```python
from build123d import *
from build123d.topology import SkipClean

# Parameters (mm, degrees)
SKETCH1_R          = 13.97
SKETCH1_R_2        = 6.604
STABILIZER_DEPTH   = 1.27
LARGE_START        = 7.9375
SKETCH2_R          = 7.366
SKETCH2_R_2        = 6.604
LARGE_END_DEPTH    = 7.9375
SMALL_START        = 7.9375
SKETCH3_R          = 7.366
SKETCH3_R_2        = 6.096
SMALL_END_DEPTH    = 7.9375
SKETCH5_W          = 3.81
SKETCH5_H          = 13.335
CUT_EXTRUDE1_DEPTH = 31.730063798
SKETCH7_W          = 3.81
SKETCH7_H          = 13.335
CUT_EXTRUDE2_DEPTH = 31.730063798


with BuildPart() as part:
    # Sketch1 → Stabilizer (new body)
    with BuildSketch(Plane(origin=(0, 0, 0), x_dir=(1, 0, 0), z_dir=(0, 1, 0))):
        with Locations(Location((0, 0, 0), (0, 0, 270))):
            Circle(SKETCH1_R)
        with Locations(Location((0, 0, 0), (0, 0, 270))):
            Circle(SKETCH1_R_2, mode=Mode.SUBTRACT)
    extrude(amount=STABILIZER_DEPTH)

    # Sketch2 → Large End (add)
    with SkipClean():  # the faces are left unmerged after this step: merging them gives an invalid solid
        with BuildSketch(Plane(origin=(0, 0, 0), x_dir=(-1, 0, 0), z_dir=(0, -1, 0)).offset(LARGE_START)):
            with Locations(Location((0, 0, 0), (0, 0, 270))):
                Circle(SKETCH2_R)
            with Locations(Location((0, 0, 0), (0, 0, 90))):
                Circle(SKETCH2_R_2, mode=Mode.SUBTRACT)
        extrude(amount=-LARGE_END_DEPTH)

    # Sketch3 → Small End (add)
    with SkipClean():  # the faces are left unmerged after this step: merging them gives an invalid solid
        with BuildSketch(Plane(origin=(0, -7.9375, 0), x_dir=(-1, 0, 0), z_dir=(0, -1, 0)).offset(SMALL_START)):
            with Locations(Location((0, 0, 0), (0, 0, 270))):
                Circle(SKETCH3_R)
            with Locations(Location((0, 0, 0), (0, 0, 90))):
                Circle(SKETCH3_R_2, mode=Mode.SUBTRACT)
        extrude(amount=-SMALL_END_DEPTH)

    # Sketch5 → Cut-Extrude1 (cut, through all)
    with SkipClean():  # the faces are left unmerged after this step: merging them gives an invalid solid
        with BuildSketch(Plane(origin=(0, -15.875, 7.366), x_dir=(1, 0, 0), z_dir=(0, 0, 1))):
            with Locations((0, 9.2075)):
                Rectangle(SKETCH5_W, SKETCH5_H)
        extrude(amount=-CUT_EXTRUDE1_DEPTH, mode=Mode.SUBTRACT)
    add(part.part.scale(1), mode=Mode.REPLACE)  # the faces are merged on a copy

    # Sketch7 → Cut-Extrude2 (cut, through all)
    with BuildSketch(Plane(origin=(7.366, -15.875, 0), x_dir=(0, 0, -1), z_dir=(1, 0, 0))):
        with Locations((0, 9.2075)):
            Rectangle(SKETCH7_W, SKETCH7_H)
    extrude(amount=-CUT_EXTRUDE2_DEPTH, mode=Mode.SUBTRACT)


solid = part.part
```
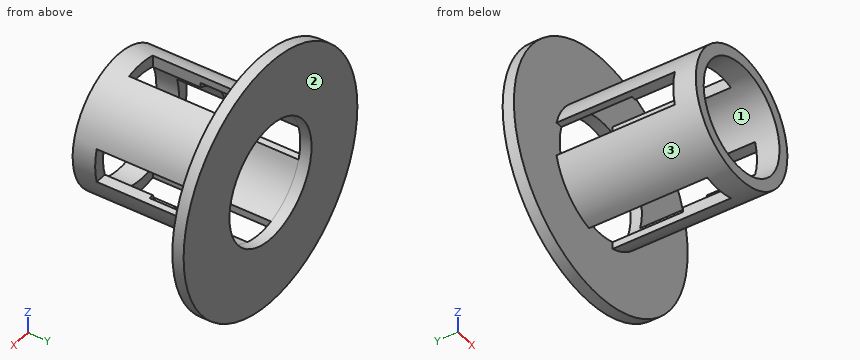
Could you check a few things on this model? Use its own coordinates, in mm. Face numbers are marked on the shaded views. Give positions to 0.01 mm unless a question says otherwise; leave off trailing zeros. Loops run counter-clockwise (first coordinate to the right, second up) from the corner with the lowest first, then second, coordinate; pieces in that order, holes last. Notation, with made-up numbers: (-7.75, 1.25) - (30.25, 1.25) arc R26 cw to (30.25, 17.25) - close; hole circle Ø2 at (-3, 17.25). An arc over 180 degrees is marked (long way). Answer in a Markdown table with one row per item. Add a question column.
Q1. If we section it at D-D (y = -14.5): List the corners of the cut face in (x, z) for me.
Q2. Please list where these lines run through material, in increasing order: L1, parallel to X at y = 1, z = 0; L2, parallel to X at y = -13.75, z = 0. Write a range as from..to.
Q3. If we section it at B-B (x = 0): List the corners of the cut face in (y, z) for me (3 decimals).
Q4. If we section it at C-C (z = 4): List the corners of the cut face in (x, y) for me (1 decimal), plus the area to 3 significant figures.
Q5. We'd pull the mould along Z, two halves only. Please class the marked faces 1, 2 and 3: +Z half, -Z half, draft (parallel to the pull), parting line (faces both ways), or undercut.
Q6. For pin 1 (0.7 mm diameter, centred on x = -6.5, y = -6.5, fed in from -Z); pin 2 (1.3 mm diameter, centred on x = 4.5, z = 4, fed in from +Y); pin 3 (0.7 mm diameter, centred on y = -6.5, z = 6, fed in from -X); pin 4 (8 mm diameter, centred on x = 0, z = 0.5, fed in from +Y), each with a flat end and sliding along its axis, tell me the tip position at first contact or that it passes through.
Q7. If we section it at A-A (y = -3.5): List the corners of the cut face in (x, z) for me (3 decimals), plus the area to 3 significant figures.
The answers:
| question | item | result |
|---|---|---|
| 1 | outline | circle Ø14.73 at (0, 0); hole circle Ø12.19 at (0, 0) |
| 2 | L1 | x = -13.97..-6.6, 6.6..13.97 |
| 2 | L2 | x = -7.37..-6.1, 6.1..7.37 |
| 3 | outline | (-15.875, -7.366) - (-13.335, -7.366) - (-13.335, -6.096) - (-15.875, -6.096) - close; (-15.875, 6.096) - (-13.335, 6.096) - (-13.335, 7.366) - (-15.875, 7.366) - close; (0, -13.97) - (1.27, -13.97) - (1.27, -6.604) - (0, -6.604) - close; (0, 6.604) - (1.27, 6.604) - (1.27, 13.97) - (0, 13.97) - close |
| 4 | outline | (-13.4, 0) - (-6.2, 0) - (-6.2, -15.9) - (-4.6, -15.9) - (-4.6, -7.9) - (-5.3, -7.9) - (-5.3, 1.3) - (-13.4, 1.3) - close; (4.6, -15.9) - (6.2, -15.9) - (6.2, 0) - (13.4, 0) - (13.4, 1.3) - (5.3, 1.3) - (5.3, -7.9) - (4.6, -7.9) - close |
| 4 | area | 60.6 mm^2 |
| 5 | face 1 | undercut |
| 5 | face 2 | draft |
| 5 | face 3 | parting line |
| 6 | pin 1 | stops at z = -4.05 |
| 6 | pin 2 | stops at y = 1.27 |
| 6 | pin 3 | stops at x = -4.73 |
| 6 | pin 4 | passes through |
| 7 | outline | (-7.115, -1.905) arc R7.366 ccw to (-1.905, -7.115) - (-1.905, -6.323) arc R6.604 cw to (-6.323, -1.905) - close; (-7.115, 1.905) - (-6.323, 1.905) arc R6.604 cw to (-1.905, 6.323) - (-1.905, 7.115) arc R7.366 ccw to start; (1.905, -7.115) arc R7.366 ccw to (7.115, -1.905) - (6.323, -1.905) arc R6.604 cw to (1.905, -6.323) - close; (1.905, 6.323) arc R6.604 cw to (6.323, 1.905) - (7.115, 1.905) arc R7.366 ccw to (1.905, 7.115) - close |
| 7 | area | 21.7 mm^2 |
